The model under review builds one solid part; all positions refer to its coordinate system, in mm. Face numbers are marked on the shaded views. A direction names the side the tool comes from. Coordinates: 2 decimals unless noted, no trailing zeros. Loops run counter-clockwise (first coordinate to the right, second up) from the corner with the lowest first, then second, coordinate; pieces in that order, holes last. Notation, with made-up numbers: M -27.5,19 L -18.5,19 A16 cw -18.5,44 Z; hole C 49.5,-2 d1. An arc over 180 degrees is marked long. Use CSV: the item, a comma, the result in double quotes. Start each with the question number.
from build123d import *

# Parameters (mm, degrees)
SKETCH1_W           = 101.6
SKETCH1_H           = 355.6
BOSS_EXTRUDE1_DEPTH = 25.4
SKETCH2_W           = 76.2
SKETCH2_H           = 25.4
BOSS_EXTRUDE2_DEPTH = 127
SKETCH3_W           = 25.4
SKETCH3_H           = 279.4
BOSS_EXTRUDE3_DEPTH = 25.4
SKETCH5_W           = 25.4
SKETCH5_H           = 279.4
BOSS_EXTRUDE4_DEPTH = 25.4
SKETCH6_W           = 25.4
SKETCH6_H           = 76.2
BOSS_EXTRUDE5_DEPTH = 50.8
SKETCH8_W           = 25.4
SKETCH8_H           = 76.2
BOSS_EXTRUDE6_DEPTH = 50.8
SKETCH9_W           = 101.6
SKETCH9_H           = 25.4
BOSS_EXTRUDE7_DEPTH = 50.8
LOFT1_DEPTH         = 101.6
CUT_EXTRUDE2_DEPTH  = 539.816024431
SKETCH18_W          = 20.6502
SKETCH18_H          = 38.1
CUT_EXTRUDE3_DEPTH  = 4.7498


# Read off the part's stored shape, not the designer's step: Loft1
with BuildPart() as part:
    # Sketch1 → Boss-Extrude1 (new body)
    with BuildSketch(Plane(origin=(0, 0, 0), x_dir=(1, 0, 0), z_dir=(0, 1, 0))):
        with Locations((50.8, 177.8)):
            Rectangle(SKETCH1_W, SKETCH1_H)
    extrude(amount=BOSS_EXTRUDE1_DEPTH)

    # Sketch2 → Boss-Extrude2 (add)
    with BuildSketch(Plane.ZY):
        with Locations((-317.5, 12.7)):
            Rectangle(SKETCH2_W, SKETCH2_H)
    extrude(amount=BOSS_EXTRUDE2_DEPTH)

    # Sketch3 → Boss-Extrude3 (add)
    with BuildSketch(Plane(origin=(0, 25.4, 0), x_dir=(1, 0, 0), z_dir=(0, 1, 0))):
        with Locations((12.7, 139.7)):
            Rectangle(SKETCH3_W, SKETCH3_H)
    extrude(amount=BOSS_EXTRUDE3_DEPTH)

    # Sketch5 → Boss-Extrude4 (add)
    with BuildSketch(Plane(origin=(0, 25.4, 0), x_dir=(1, 0, 0), z_dir=(0, 1, 0))):
        with Locations((88.9, 139.7)):
            Rectangle(SKETCH5_W, SKETCH5_H)
    extrude(amount=BOSS_EXTRUDE4_DEPTH)

    # Sketch6 → Boss-Extrude5 (add)
    with BuildSketch(Plane(origin=(0, 50.8, 0), x_dir=(1, 0, 0), z_dir=(0, 1, 0))):
        with Locations((12.7, 139.7)):
            Rectangle(SKETCH6_W, SKETCH6_H)
    extrude(amount=BOSS_EXTRUDE5_DEPTH)

    # Sketch8 → Boss-Extrude6 (add)
    with BuildSketch(Plane(origin=(0, 50.8, 0), x_dir=(1, 0, 0), z_dir=(0, 1, 0))):
        with Locations((88.9, 139.7)):
            Rectangle(SKETCH8_W, SKETCH8_H)
    extrude(amount=BOSS_EXTRUDE6_DEPTH)

    # Sketch9 → Boss-Extrude7 (add)
    with BuildSketch(Plane(origin=(0, 0, -355.6), x_dir=(-1, 0, 0), z_dir=(0, 0, -1))):
        with Locations((-50.8, 12.7)):
            Rectangle(SKETCH9_W, SKETCH9_H)
    extrude(amount=BOSS_EXTRUDE7_DEPTH)

    # Loft1 outline → Loft1 (add)
    with BuildSketch(Plane.YZ):
        Polygon((25.4, -406.4), (152.4, -508.000697031), (152.4, -457.200697031), (25.4, -355.6), align=None)
    extrude(amount=LOFT1_DEPTH)

    # Sketch17 → Cut-Extrude2 (cut, through all)
    with BuildSketch(Plane(origin=(0, 25.4, 0), x_dir=(1, 0, 0), z_dir=(0, 1, 0))):
        Polygon((101.6, 304.8), (101.6, 330.2), (76.128136844, 339.471), (76.128136844, 295.529), align=None)
    extrude(amount=-CUT_EXTRUDE2_DEPTH, mode=Mode.SUBTRACT)

    # Sketch18 → Cut-Extrude3 (cut)
    with BuildSketch(Plane(origin=(0, 101.6, 0), x_dir=(1, 0, 0), z_dir=(0, 1, 0))):
        with Locations((10.3251, 139.7)):
            Rectangle(SKETCH18_W, SKETCH18_H)
    extrude(amount=-CUT_EXTRUDE3_DEPTH, mode=Mode.SUBTRACT)


solid = part.part
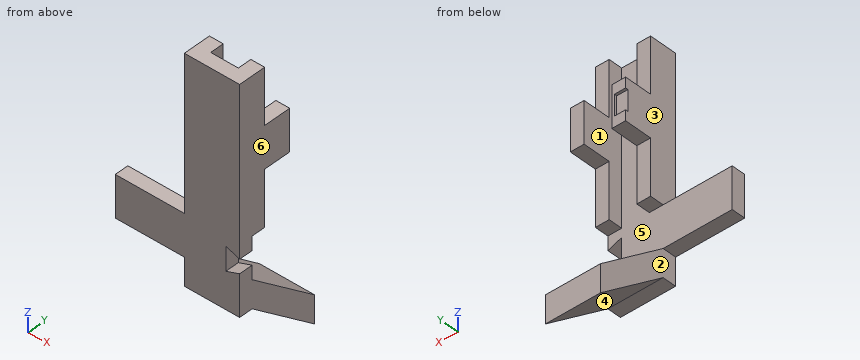
1. For the marked faces 1, 2 and 3, list the 3-axis set-ups (+Z, -Z, +X, -X, +Y, -Y) from which the entire face can be reached by the end or side of a thin tool; tool diameter is ignored.
2. Insertion check: pin 1 Ø12.5 at (x, y) = (-93.5, 11.5) entering from +Z; pin 2 Ø12.5 at (x, z) = (14.5, -35.5) entering from +Y; pin 3 Ø12.5 at (x, y) = (95, 35.5) entering from -Z. Each pin has a flat end and moves straight along its axis. Give the tip position at first contact, or say it passes through.
3. Add section A-A (z = -232). Write out the cut boundary in (x, y), plus the area to 3 significant figures.
4. To check wall thickness, follow line 1 along X through (y, z) = (47, -31.5); line 2 along Y through (x, z) = (57.5, -71); line 3 along X through (y, z) = (80, -409.5). State the ranges of each line that lie inside material, in increasing order.
5. Draft analysis for pull direction X (two halves, no side actions). For the marked faces 4, 5 and 6, state which applies: released by +X, released by -X, zero draft, split by the parting line, or undercut.
6. Add section C-C (y = 16). Write out the cut boundary in (x, z).
7. Add section D-D (y = 65.5). Write out the cut boundary in (x, z), plus the area to 3 significant figures.
8. Add section B-B (x = 5). Write out the cut boundary in (y, z), plus the area to 3 significant figures.
Solved:
1,face 1,"+Z, +Y"
1,face 2,"-Z, -X, +Y, -Y"
1,face 3,"+Z, -X, +Y, -Y"
2,pin 1,"stops at z = -279.4"
2,pin 2,"stops at y = 50.8"
2,pin 3,"stops at z = -419.48"
3,outline,"M 0,0 L 101.6,0 L 101.6,50.8 L 76.2,50.8 L 76.2,25.4 L 25.4,25.4 L 25.4,50.8 L 0,50.8 Z"
3,area,"3,870 mm^2"
4,line 1,"x = 0 to 25.4, 76.2 to 101.6"
4,line 2,"y = 0 to 25.4"
4,line 3,"x = 0 to 101.6"
5,face 4,"zero draft"
5,face 5,"undercut"
5,face 6,"released by +X"
6,outline,"M -127,-355.6 L 0,-355.6 L 0,-406.4 L 101.6,-406.4 L 101.6,-330.2 L 76.13,-339.47 L 76.13,-295.53 L 101.6,-304.8 L 101.6,0 L 0,0 L 0,-279.4 L -127,-279.4 Z"
7,outline,"M 0,-438.48 L 101.6,-438.48 L 101.6,-387.68 L 0,-387.68 Z; M 0,-177.8 L 25.4,-177.8 L 25.4,-101.6 L 0,-101.6 Z; M 76.2,-177.8 L 101.6,-177.8 L 101.6,-101.6 L 76.2,-101.6 Z"
7,area,"9,030 mm^2"
8,outline,"M 0,-406.4 L 25.4,-406.4 L 152.4,-508 L 152.4,-457.2 L 25.4,-355.6 L 25.4,-279.4 L 50.8,-279.4 L 50.8,-177.8 L 101.6,-177.8 L 101.6,-158.75 L 96.85,-158.75 L 96.85,-120.65 L 101.6,-120.65 L 101.6,-101.6 L 50.8,-101.6 L 50.8,0 L 0,0 Z"
8,area,"27,600 mm^2"
